The listing builds one solid part. Answer for the finished solid, in the listing's coordinates (mm). A direction names the side the tool comes from. Round coordinates to 2 decimals unless told otherwise and drop trailing zeros. Write each loop counter-clockwise with the first axis right and the second up, starting at its lowest first coordinate (ties: lowest second). Pieces come first, ordered by that corner, then holes. Notation, with made-up numbers: (21.25, 13) - (64.25, 13) arc R29 cw to (64.25, 36) - close; hole circle Ø9 at (62, 77.25). An arc over 180 degrees is marked (long way). Return JSON: item names as keys, results as strings. Group by question number.
from build123d import *

# Parameters (mm, degrees)
BOSS_EXTRUDE1_DEPTH = 4
SKETCH2_R           = 1.5
BOSS_EXTRUDE2_DEPTH = 4
FILLET1_DEPTH       = 4


with BuildPart() as part:
    # Sketch1 → Boss-Extrude1 (new body)
    with BuildSketch(Plane.XY):
        Polygon((-70, -65.358547654), (-14.572335871, -45.184527756), (-14.572335871, -47.312883301), (-70, -67.486903199), align=None)
    extrude(amount=BOSS_EXTRUDE1_DEPTH)

    # Sketch2 → Boss-Extrude2 (add)
    # profile 1 of 6: a face of its own
    with BuildSketch(Plane(origin=(0, 0, 0), x_dir=(-1, 0, 0), z_dir=(0, 0, -1))):
        with BuildLine():
            ThreePointArc((15.753480329, -49.871140271), (17.845334, -54.357134945), (22.331328674, -52.265281274))
            ThreePointArc((22.331328674, -52.265281274), (22.489231637, -51.675979394), (22.542404501, -51.068210772))
            ThreePointArc((22.542404501, -51.068210772), (22.513056924, -50.615914674), (22.425506352, -50.171203601))
            Line((22.425506352, -50.171203601), (17.027383224, -48.206447461))
            ThreePointArc((17.027383224, -48.206447461), (16.262879385, -48.941184649), (15.753480329, -49.871140271))
        make_face()
        with Locations((19.042404501, -51.068210772)):
            Circle(SKETCH2_R, mode=Mode.SUBTRACT)
    # profile 2 of 6: a face of its own
    with BuildSketch(Plane(origin=(0, 0, 0), x_dir=(-1, 0, 0), z_dir=(0, 0, -1))):
        with BuildLine():
            Line((16.437520615, -47.991755029), (15.753480329, -49.871140271))
            ThreePointArc((15.753480329, -49.871140271), (16.262879385, -48.941184649), (17.027383224, -48.206447461))
            Line((17.027383224, -48.206447461), (16.437520615, -47.991755029))
        make_face()
    # profile 3 of 6: a face of its own
    with BuildSketch(Plane(origin=(0, 0, 0), x_dir=(-1, 0, 0), z_dir=(0, 0, -1))):
        with BuildLine():
            Line((22.331328674, -52.265281274), (23.015368961, -50.385896032))
            Line((23.015368961, -50.385896032), (22.425506352, -50.171203601))
            ThreePointArc((22.425506352, -50.171203601), (22.513056924, -50.615914674), (22.542404501, -51.068210772))
            ThreePointArc((22.542404501, -51.068210772), (22.489231637, -51.675979394), (22.331328674, -52.265281274))
        make_face()
    # profile 4 of 6: a face of its own
    with BuildSketch(Plane(origin=(0, 0, 0), x_dir=(-1, 0, 0), z_dir=(0, 0, -1))):
        with BuildLine():
            ThreePointArc((62.132629021, -64.62341434), (61.368125183, -65.358151529), (60.858726126, -66.28810715))
            ThreePointArc((60.858726126, -66.28810715), (62.950579797, -70.774101825), (67.436574472, -68.682248154))
            ThreePointArc((67.436574472, -68.682248154), (67.594477435, -68.092946274), (67.647650299, -67.485177652))
            ThreePointArc((67.647650299, -67.485177652), (67.618302722, -67.032881553), (67.53075215, -66.58817048))
            Line((67.53075215, -66.58817048), (62.132629021, -64.62341434))
        make_face()
        with Locations((64.147650299, -67.485177652)):
            Circle(SKETCH2_R, mode=Mode.SUBTRACT)
    # profile 5 of 6: a face of its own
    with BuildSketch(Plane(origin=(0, 0, 0), x_dir=(-1, 0, 0), z_dir=(0, 0, -1))):
        with BuildLine():
            Line((62.132629021, -64.62341434), (61.542766413, -64.408721909))
            Line((61.542766413, -64.408721909), (60.858726126, -66.28810715))
            ThreePointArc((60.858726126, -66.28810715), (61.368125183, -65.358151529), (62.132629021, -64.62341434))
        make_face()
    # profile 6 of 6: a face of its own
    with BuildSketch(Plane(origin=(0, 0, 0), x_dir=(-1, 0, 0), z_dir=(0, 0, -1))):
        with BuildLine():
            ThreePointArc((67.647650299, -67.485177652), (67.594477435, -68.092946274), (67.436574472, -68.682248154))
            Line((67.436574472, -68.682248154), (68.120614758, -66.802862912))
            Line((68.120614758, -66.802862912), (67.53075215, -66.58817048))
            ThreePointArc((67.53075215, -66.58817048), (67.618302722, -67.032881553), (67.647650299, -67.485177652))
        make_face()
    extrude(amount=-BOSS_EXTRUDE2_DEPTH)

    # Fillet1: read off the stored shape, not the designer's step
    # Fillet1 outline → Fillet1 (add)
    with BuildSketch(Plane.XY):
        with BuildLine():
            ThreePointArc((-15.753480329, -49.871140271), (-15.583589929, -50.532858787), (-15.545482945, -51.214974613))
            ThreePointArc((-15.545482945, -51.214974613), (-15.257091898, -49.214503996), (-14.572335871, -47.312883301))
            Line((-14.572335871, -47.312883301), (-16.437520615, -47.991755029))
            Line((-16.437520615, -47.991755029), (-15.753480329, -49.871140271))
        make_face()
        with BuildLine():
            Line((-23.015368961, -50.385896032), (-29.94492695, -52.908048877))
            ThreePointArc((-29.94492695, -52.908048877), (-25.335591086, -52.375928842), (-20.982265505, -53.981445964))
            ThreePointArc((-20.982265505, -53.981445964), (-21.794013834, -53.231228591), (-22.331328674, -52.265281274))
            Line((-22.331328674, -52.265281274), (-23.015368961, -50.385896032))
        make_face()
        with BuildLine():
            ThreePointArc((-60.858726126, -66.28810715), (-60.649434207, -67.373445046), (-60.78903907, -68.469926664))
            ThreePointArc((-60.78903907, -68.469926664), (-58.486204715, -64.44176545), (-54.613208423, -61.886569064))
            Line((-54.613208423, -61.886569064), (-61.542766413, -64.408721909))
            Line((-61.542766413, -64.408721909), (-60.858726126, -66.28810715))
        make_face()
        with BuildLine():
            ThreePointArc((-70, -67.486903199), (-68.243205646, -68.501846695), (-66.727429559, -69.850497708))
            ThreePointArc((-66.727429559, -69.850497708), (-67.139576393, -69.301321437), (-67.436574472, -68.682248154))
            Line((-67.436574472, -68.682248154), (-68.120614758, -66.802862912))
            Line((-68.120614758, -66.802862912), (-70, -67.486903199))
        make_face()
    extrude(amount=FILLET1_DEPTH)


solid = part.part
(1) For faces 4 (the flat face through (-42, -57, 0)), 5 (the flat face through (-42.106, -57.334, 1.972)), determine the directions among +Z, -Z, +X, -X, +Y, -Y from which every point of the face is accessible in a straight line to the end or side of a thin tool.
(2) A flat-ended cylindrical pin translates along its axis: pin 1 (2 mm diameter, centred on x = -43, z = 1.5, fed in from +Y). Find the tip coordinate at first contact, or state that the pin passes through.
(3) Find section B-B (x = -27). Write down the section's boundary in (y, z).
(4) Find section A-A (z = 1.2). Write down the section's boundary in (x, y).
(5) Find section C-C (y = -56.5). Write down the section's boundary in (x, z).
(6) Determine the mould class of faces 1 (the cylindrical face through (-17.409, -54.164, 1.972)), 2 (the cylindrical face through (-58.53, -64.49, 1.97)), 3 (the cylindrical face through (-63.3, -70.88, 1.97)) for opening direction X: +X half, -X half, draft (parallel to the pull), parting line (faces both ways), or undercut.
(7) Consider line 1 (Y direction, x = -18, z = 3.65); line 2 (Y direction, x = -59, z = 3.75); line 3 (Y direction, x = -55.5, z = 2.05). Determine where each line is inside the solid, lowest interval first.
Check sheet entries:
{
 "1": {"face 4": "-Z, +X, -X, +Y, -Y", "face 5": "+Z, -Z, -Y"},
 "2": {"pin 1": "stops at y = -55.17"},
 "3": {"outline": "(-52.32, 0) - (-49.71, 0) - (-49.71, 4) - (-52.32, 4) - close"},
 "4": {"outline": "(-70, -67.49) arc R10 cw to (-66.73, -69.85) arc R3.5 ccw to (-60.79, -68.47) arc R10 cw to (-54.61, -61.89) - (-29.94, -52.91) arc R10 cw to (-20.98, -53.98) arc R3.5 ccw to (-15.55, -51.21) arc R10 cw to (-14.57, -47.31) - (-14.57, -45.18) - (-70, -65.36) - close; hole circle Ø3 at (-64.15, -67.49); hole circle Ø3 at (-19.04, -51.07)"},
 "5": {"outline": "(-45.66, 0) - (-39.81, 0) - (-39.81, 4) - (-45.66, 4) - close"},
 "6": {"face 1": "undercut", "face 2": "+X half", "face 3": "parting line"},
 "7": {"line 1": "y = -54.41 to -52.15, -49.99 to -46.43", "line 2": "y = -65.03 to -61.35", "line 3": "y = -62.26 to -60.08"}
}
